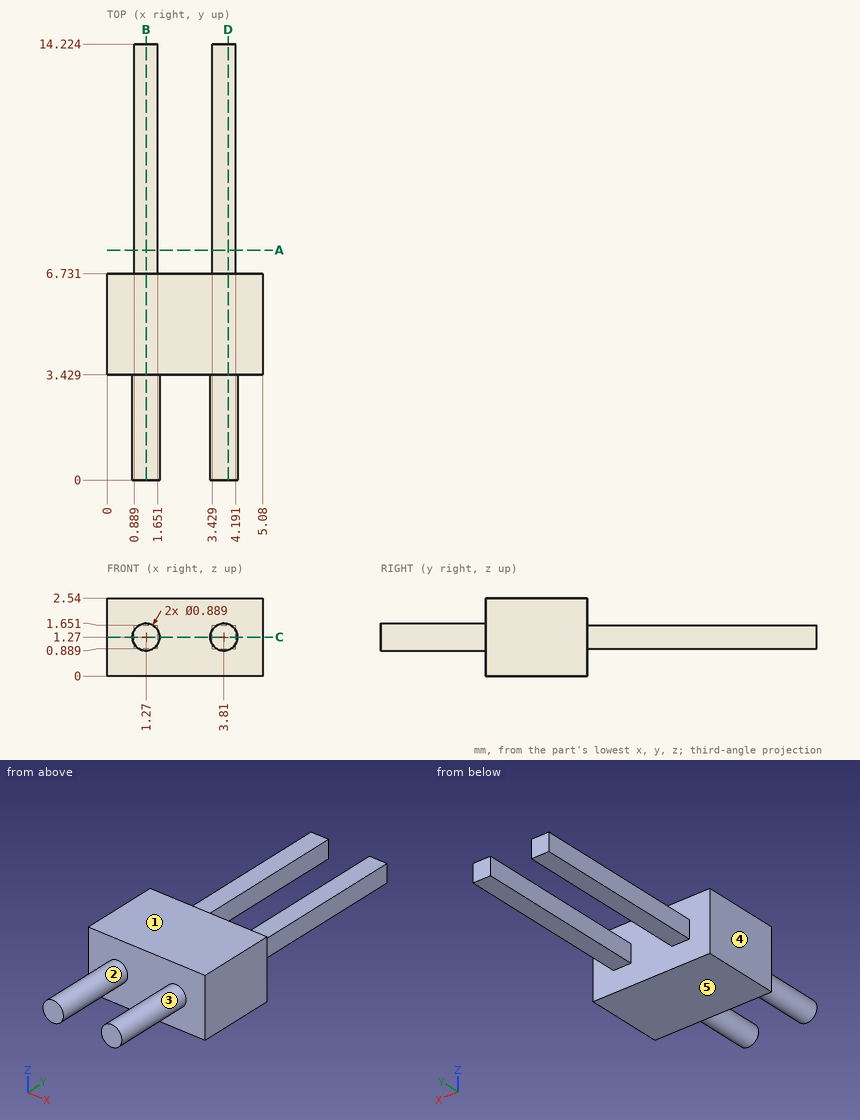
Print and shaded views of the part. All mm, measured from the part's lowest x, y and z. A direction names the side the tool comes from. Coordinates: 2 decimals unless noted, no trailing zeros. Order: outer loops, then holes, each group sorted by start corner. A loop starts at its lowest first (then second) coordinate and runs counter-clockwise, first axis right, second up. Notation, with made-up numbers: (12.25, 44) -> (22.25, 44) arc R20 cw to (22.25, 57) -> close; hole circle Ø5 at (-3.5, -35.75). An arc over 180 degrees is marked (long way). Use one line per item in the form item = value. Start each with the question number.
1) Band-saw the part on C-C on z = 1.27. Give the cut face in (x, y), then the cut area to 3 significant figures.
2) Band-saw the part on A-A on y = 7.5. Give the cut face in (x, z), then the cut area to 3 significant figures.
3) Band-saw the part on D-D on x = 3.95. Give the cut face in (y, z).
4) Pull direction X, two halves, no side cores. Call the marked faces 3, 4 and 5: +X half, -X half, draft (parallel to the pull), parting line (faces both ways), or undercut.
5) Drop flat-ended pins along their axis: pin 1 (1 mm diameter, centred on y = 6, z = 1, fed in from -X); pin 2 (0.8 mm diameter, centred on y = 9.5, z = 1, fed in from +X); pin 3 (0.8 mm diameter, centred on y = 9, z = 1.5, fed in from -X); pin 4 (0.8 mm diameter, centred on x = 1, y = 9, fed in from +Z). Give the stop position or say it passes through.
6) Drill centre lines: L1, parallel to X at y = 11, z = 1.55; L2, parallel to Z at x = 4, y = 13.5; L3, parallel to Y at x = 3.3, z = 1.6. Where is each one in solid material? Low to high. Write a range as [from, to].
7) Tool access for the marked faces 1 and 2: list every direction of +Z, -Z, +X, -X, +Y, -Y with a clear straight run to the whole face (end or side of a thin tool).
8) Band-saw the part on B-B on x = 1.27. Give the cut face in (y, z).
Entries:
q1.outline = (0, 3.43) -> (0.83, 3.43) -> (0.83, 0) -> (1.71, 0) -> (1.71, 3.43) -> (3.37, 3.43) -> (3.37, 0) -> (4.25, 0) -> (4.25, 3.43) -> (5.08, 3.43) -> (5.08, 6.73) -> (4.19, 6.73) -> (4.19, 14.22) -> (3.43, 14.22) -> (3.43, 6.73) -> (1.65, 6.73) -> (1.65, 14.22) -> (0.89, 14.22) -> (0.89, 6.73) -> (0, 6.73) -> close
q1.area = 34.3 mm2
q2.outline = (0.89, 0.89) -> (1.65, 0.89) -> (1.65, 1.65) -> (0.89, 1.65) -> close; (3.43, 0.89) -> (4.19, 0.89) -> (4.19, 1.65) -> (3.43, 1.65) -> close
q2.area = 1.16 mm2
q3.outline = (0, 0.85) -> (3.43, 0.85) -> (3.43, 0) -> (6.73, 0) -> (6.73, 0.89) -> (14.22, 0.89) -> (14.22, 1.65) -> (6.73, 1.65) -> (6.73, 2.54) -> (3.43, 2.54) -> (3.43, 1.69) -> (0, 1.69) -> close
q4.face_3 = undercut
q4.face_4 = -X half
q4.face_5 = draft
q5.pin_1 = 0
q5.pin_2 = 4.19
q5.pin_3 = 0.89
q5.pin_4 = 1.65
q6.L1 = [0.89, 1.65], [3.43, 4.19]
q6.L2 = [0.89, 1.65]
q6.L3 = [3.43, 6.73]
q7.face_1 = +Z, +X, -X, +Y, -Y
q7.face_2 = -Y
q8.outline = (0, 0.83) -> (3.43, 0.83) -> (3.43, 0) -> (6.73, 0) -> (6.73, 0.89) -> (14.22, 0.89) -> (14.22, 1.65) -> (6.73, 1.65) -> (6.73, 2.54) -> (3.43, 2.54) -> (3.43, 1.71) -> (0, 1.71) -> close
